```python
from build123d import *

# Parameters (mm, degrees)
ESTRUSIONE_ESTRUSIONE1_DEPTH = 60


with BuildPart() as part:
    # Schizzo1 → Estrusione-Estrusione1 (new body)
    with BuildSketch(Plane.XY):
        with BuildLine():
            Line((0, 0), (96, 0))
            Line((96, 0), (96, 12.398749749))
            Line((96, 12.398749749), (92, 12.398749749))
            ThreePointArc((92, 12.398749749), (90.398749749, 14), (92, 15.601250251))
            Line((92, 15.601250251), (96, 15.601250251))
            Line((96, 15.601250251), (96, 25))
            Line((96, 25), (0, 25))
            Line((0, 25), (0, 15.601250251))
            Line((0, 15.601250251), (4, 15.601250251))
            ThreePointArc((4, 15.601250251), (5.601250251, 14), (4, 12.398749749))
            Line((4, 12.398749749), (0, 12.398749749))
            Line((0, 12.398749749), (0, 0))
        make_face()
    extrude(amount=ESTRUSIONE_ESTRUSIONE1_DEPTH)


solid = part.part
```
Check sheet for the modelled part. Datum: model origin and axes. Units: mm. A direction names the side the tool comes from. Coordinates: 2 decimals unless noted, no trailing zeros. Order: outer loops, then holes, each group sorted by start corner. A loop starts at its lowest first (then second) coordinate and runs counter-clockwise, first axis right, second up. Notation, with made-up numbers: (-7, -37) -> (0, -37) arc R20 cw to (0, -15) -> close; hole circle Ø7 at (73.25, 37). An arc over 180 degrees is marked (long way). Write each question's results on one line, items separated by ' | '. Start each with the question number.
1) Material ranges on line 1 along X through (y, z) = (14.75, 52); line 2 along X through (y, z) = (14.5, 26.5), recorded low to high.
2) Section check A-A (y = 14). Enter the section's corners in (x, z).
3) Set-up check for faces 1 (the face through (2, 15.601, 30)), 2 (the face through (47, 13, 60)), 3 (the face through (94, 15.601, 30)): record each of +Z, -Z, +X, -X, +Y, -Y from which the full face is reachable in a straight line by a thin tool's end or side.
4) Draft check along Y on faces 4 (the face through (49, 25, 30)), 5 (the face through (47, 0, 30)), 6 (the face through (96, 6, 30)), 7 (the face through (94, 12.399, 30)). Enter one of: pulls with the +Y half, pulls with the -Y half, needs draft (parallel to the pull), parting line crosses it, or undercut.
Checked values:
1) line 1: 5.41 to 90.59 | line 2: 5.52 to 90.48
2) outline: (5.6, 0) -> (90.4, 0) -> (90.4, 60) -> (5.6, 60) -> close
3) face 1: +Z, -Z, -X | face 2: +Z, +X, -X, +Y, -Y | face 3: +Z, -Z, +X
4) face 4: pulls with the +Y half | face 5: pulls with the -Y half | face 6: needs draft | face 7: undercut
